For this review, take the finished solid that the model builds, in its own axes (mm). Coordinates: 2 decimals unless noted, no trailing zeros. Loops run counter-clockwise (first coordinate to the right, second up) from the corner with the lowest first, then second, coordinate; pieces in that order, holes last. Notation, with made-up numbers: M 20.25,-16 L 52.25,-16 A10 cw 52.25,-8 Z; hole C 74.25,30.25 d9. An arc over 180 degrees is marked long. Write item = value, one per line.
from build123d import *

# Parameters (mm, degrees)
F0_W     = 44.45
F0_H     = 44.45
F0_R     = 15.875
F1_DEPTH = 20.32
F3_DEPTH = 20.321


with BuildPart() as f1:
    # F0 (on Top) → F1 (new body)
    with BuildSketch(Plane.XY):
        Rectangle(F0_W, F0_H)
        Circle(F0_R, mode=Mode.SUBTRACT)
    extrude(amount=F1_DEPTH)

    # F2 (on face) → F3 (cut, through all)
    with BuildSketch(Plane.XY.offset(20.32)):
        with BuildLine():
            Line((-22.225, -13.335), (-22.225, -22.225))
            Line((-22.225, -22.225), (22.225, -22.225))
            Line((22.225, -22.225), (22.225, -13.335))
            Line((22.225, -13.335), (8.613559, -13.335))
            ThreePointArc((8.613559, -13.335), (0, -15.875), (-8.613559, -13.335))
            Line((-8.613559, -13.335), (-22.225, -13.335))
        make_face()
    extrude(amount=-F3_DEPTH, mode=Mode.SUBTRACT)


solid = f1.part
Q1. For line 1 along X through (y, z) = (0, 4.5) (3 decimals); line 2 along X through (y, z) = (-10, 13) (3 decimals); line 3 along Y through (x, z) = (0, 6.75) (3 decimals), list the stretches that pass through material, from the lowest coordinate up.
Solved:
line_1 = -22.225 to -15.875, 15.875 to 22.225
line_2 = -22.225 to -12.329, 12.329 to 22.225
line_3 = 15.875 to 22.225
Q2. Add section A-A (x = 14). Write out the cut boundary in (y, z) (3 decimals), and give its area (3 significant figures).
Solved:
outline = M -13.335,0 L -7.484,0 L -7.484,20.32 L -13.335,20.32 Z; M 7.484,0 L 22.225,0 L 22.225,20.32 L 7.484,20.32 Z
area = 418 mm²
Q3. For pin 1 Ø2 at (x, z) = (3.5, 15) entering from -Y, flat-tipped, find the tip position at first contact; note if it passes through.
Solved:
pin_1 = 15.22
Q4. Add section B-B (y = 0). Write out the cut boundary in (x, z) (3 decimals).
Solved:
outline = M -22.225,0 L -15.875,0 L -15.875,20.32 L -22.225,20.32 Z; M 15.875,0 L 22.225,0 L 22.225,20.32 L 15.875,20.32 Z
Q5. Draft analysis for pull direction Y (two halves, no side actions). For faces 1 (the face through (-15, -13.335, 10)), 2 (the face through (0, 22.225, 10)), 3 (the face through (0, 17, 0)), 4 (the face through (0.571, 15.865, 10.018)), state which applies: +Y half, -Y half, draft (parallel to the pull), parting line (faces both ways), or undercut.
Solved:
face_1 = -Y half
face_2 = +Y half
face_3 = draft
face_4 = undercut
Q6. Add section C-C (z = 7). Write out the cut boundary in (x, y) (3 decimals).
Solved:
outline = M -22.225,-13.335 L -8.614,-13.335 A15.875 cw long 8.614,-13.335 L 22.225,-13.335 L 22.225,22.225 L -22.225,22.225 Z
Q7. Add section D-D (x = 0). Write out the cut boundary in (y, z) (3 decimals), and give its area (3 significant figures).
Solved:
outline = M 15.875,0 L 22.225,0 L 22.225,20.32 L 15.875,20.32 Z
area = 129 mm²
